For this review, take the finished solid that the model builds, in its own axes (mm). Face numbers are marked on the shaded views. A direction names the side the tool comes from. Give positions to 0.01 mm unless a question says otherwise; leave off trailing zeros. Write each loop counter-clockwise with the first axis right and the second up, starting at its lowest first coordinate (ties: lowest second). Pieces come first, ordered by that corner, then holes.
1) Wall thickness on line 1 along X through (y, z) = (-14.5, 2.75) (3 decimals); line 2 along Z through (x, y) = (5, 0) (3 decimals); line 3 along Y through (x, z) = (-5, 6.35) (3 decimals): over which ranges is each line inside the solid? List them lowest first.
2) We need section C-C on x = 20. Give the boundary of the cut face in (y, z) (3 decimals), and give its area (3 significant figures).
3) Draft analysis for pull direction X (two halves, no side actions). For the marked faces 1, 2 and 3, state which applies: pulls with the +X half, pulls with the -X half, needs draft (parallel to the pull), parting line crosses it, or undercut.
4) Machinability: for the marked faces 4, 5 and 6, which of the approach directions +Z, -Z, +X, -X, +Y, -Y give a long, thin tool a straight path to every point of the face, cutting with its end or side? Answer none if there is none.
5) For P1, Ø3, axis at x = -1, z = 6, coming from the +Y side; P2, Ø4, axis at y = 0, z = 6.35, coming from the +X side; P3, Ø4, axis at x = 2.5, z = 8.5, coming from the -Y side; P4, Ø3, axis at y = 1.5, z = 11, coming from the -X side, all flat-tipped, find the tip position at first contact; note any pin that passes through.
6) We need section B-B on y = -8.5. Give the boundary of the cut face in (x, z) (3 decimals), and give its area (3 significant figures).
7) We need section A-A on z = 6.35. Give the boundary of the cut face in (x, y) (3 decimals), and give its area (3 significant figures).
8) We need section D-D on x = 0. Give the boundary of the cut face in (y, z) (3 decimals).
from build123d import *

# Parameters (mm, degrees)
F1_DEPTH       = 12.7
F3_D           = 6.35
F3_CSINK_D     = 12.7
F3_CSINK_ANGLE = 90


with BuildPart() as f1:
    # F0 (on Top) → F1 (new body)
    with BuildSketch(Plane.XY):
        Polygon((-9.525, 27.659873), (-25.4, 27.659873), (-25.4, -27.659873), (-9.525, -27.659873), (-9.525, -6.278621), (0, -6.278621), (0, 6.278621), (-9.525, 6.278621), align=None)
        Polygon((25.4, 27.659873), (9.525, 27.659873), (9.525, 6.278621), (0, 6.278621), (0, -6.278621), (9.525, -6.278621), (9.525, -27.659873), (25.4, -27.659873), align=None)
    extrude(amount=F1_DEPTH)

    # F3 (through all)
    with Locations(Plane(origin=(-25.4, 0, 0), x_dir=(0, -1, 0), z_dir=(-1, 0, 0))):
        with Locations((0, 6.35)):
            CounterSinkHole(F3_D / 2, F3_CSINK_D / 2, counter_sink_angle=F3_CSINK_ANGLE)


solid = f1.part
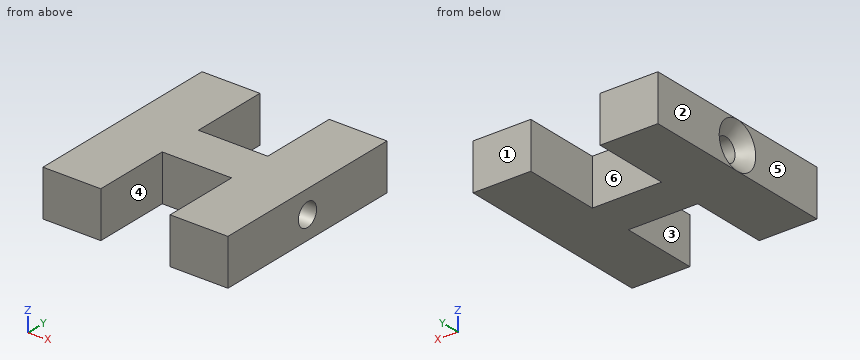
Results list:
1. line 1: x = -25.4 to -9.525, 9.525 to 25.4
1. line 2: z = 0 to 3.175, 9.525 to 12.7
1. line 3: y = -6.279 to -3.175, 3.175 to 6.279
2. outline: (-27.66, 0) - (27.66, 0) - (27.66, 12.7) - (-27.66, 12.7) - close; hole circle Ø6.35 at (0, 6.35)
2. area: 671 mm2
3. face 1: needs draft
3. face 2: pulls with the -X half
3. face 3: undercut
4. face 4: +Z, -Z, -Y
4. face 5: +Z, -Z, -X, +Y, -Y
4. face 6: +Z, -Z, +Y
5. P1: stops at y = 6.28
5. P2: passes through
5. P3: stops at y = -6.28
5. P4: stops at x = -25.4
6. outline: (-25.4, 0) - (-9.525, 0) - (-9.525, 12.7) - (-25.4, 12.7) - close; (9.525, 0) - (25.4, 0) - (25.4, 12.7) - (9.525, 12.7) - close
6. area: 403 mm2
7. outline: (-25.4, -27.66) - (-9.525, -27.66) - (-9.525, -6.279) - (9.525, -6.279) - (9.525, -27.66) - (25.4, -27.66) - (25.4, -3.175) - (-22.225, -3.175) - (-25.4, -6.35) - close; (-25.4, 6.35) - (-22.225, 3.175) - (25.4, 3.175) - (25.4, 27.66) - (9.525, 27.66) - (9.525, 6.279) - (-9.525, 6.279) - (-9.525, 27.66) - (-25.4, 27.66) - close
7. area: 1,660 mm2
8. outline: (-6.279, 0) - (6.279, 0) - (6.279, 12.7) - (-6.279, 12.7) - close; hole circle Ø6.35 at (0, 6.35)
